Source: three-view drawing plus pictorial views. Frame: mm from the lowest corner of the part. Round coordinates to 2 decimals unless told otherwise and drop trailing zeros. Order: outer loops, then holes, each group sorted by start corner. A loop starts at its lowest first (then second) coordinate and runs counter-clockwise, first axis right, second up. Notation, with made-up numbers: (55.25, 56) -> (73.25, 56) arc R25 ccw to (73.25, 77) -> close; hole circle Ø1 at (33.25, 34.5). An arc over 180 degrees is marked (long way). Answer as CSV lines item,"result".
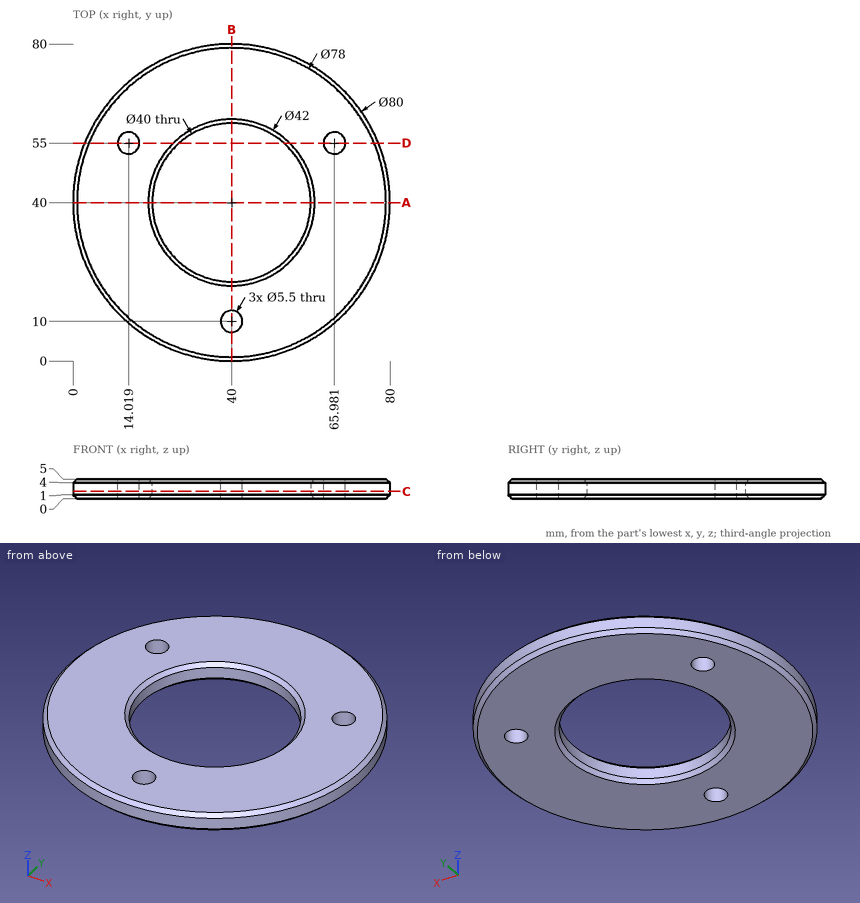
1. Line query: L1, parallel to X at y = 55, z = 2.5; L2, parallel to Y at x = 40, z = 3.35; L3, parallel to X at y = 40.5, z = 3.85. Output: solid intervals per line, ascending. Write a range as [from, to].
Results below:
L1,"[2.92, 11.27], [16.77, 26.77], [53.23, 63.23], [68.73, 77.08]"
L2,"[0, 7.25], [12.75, 20], [60, 80]"
L3,"[0, 20.01], [59.99, 80]"
2. Section query D-D on y = 55. Give the number of separate pieces and of enclosed holes in the cut face, and give its area (3 significant figures).
Results below:
separate pieces,"4"
enclosed holes,"0"
area,"178 mm2"
3. Section query C-C on z = 1.9. Return loops of the section in (x, y), and give its area (3 significant figures).
Results below:
outline,"circle Ø80 at (40, 40); hole circle Ø5.5 at (14.02, 55); hole circle Ø40 at (40, 40); hole circle Ø5.5 at (40, 10); hole circle Ø5.5 at (65.98, 55)"
area,"3,700 mm2"
4. Pin query (flat end, axial travel): pin 1 (24 mm diameter, centred on x = 40, y = 40, fed in from -Z); pin 2 (2 mm diameter, centred on x = 13, z = 1.5, fed in from +Y); pin 3 (6 mm diameter, centred on x = 53, y = 8.5, fed in from -Z); pin 4 (1 mm diameter, centred on y = 59, z = 4.5, fed in from -X). Return the tip coordinate at first contact, or that it passes through.
Results below:
pin 1,"through"
pin 2,"y = 70.4"
pin 3,"z = 0"
pin 4,"x = 4.74"
5. Section query A-A on y = 40. Return loops of the section in (x, z), and give its area (3 significant figures).
Results below:
outline,"(0, 1) -> (1, 0) -> (19, 0) -> (20, 1) -> (20, 4) -> (19, 5) -> (1, 5) -> (0, 4) -> close; (60, 1) -> (61, 0) -> (79, 0) -> (80, 1) -> (80, 4) -> (79, 5) -> (61, 5) -> (60, 4) -> close"
area,"196 mm2"
6. Section query B-B on x = 40. Return loops of the section in (y, z).
Results below:
outline,"(0, 1) -> (1, 0) -> (7.25, 0) -> (7.25, 5) -> (1, 5) -> (0, 4) -> close; (12.75, 0) -> (19, 0) -> (20, 1) -> (20, 4) -> (19, 5) -> (12.75, 5) -> close; (60, 1) -> (61, 0) -> (79, 0) -> (80, 1) -> (80, 4) -> (79, 5) -> (61, 5) -> (60, 4) -> close"
